The listing builds one solid part. Answer for the finished solid, in the listing's coordinates (mm). A direction names the side the tool comes from. Round coordinates to 2 decimals unless told otherwise and drop trailing zeros. Write each loop counter-clockwise with the first axis right and the second up, starting at its lowest first coordinate (ties: lowest second). Pieces come first, ordered by that corner, then holes. Notation, with made-up numbers: M -11.75,-35 L 46.25,-35 A15 ccw 46.25,-16 Z; hole C 50.5,30 d7. An arc over 180 degrees is marked long. Put each result on its own line as item: value. Start each with the question number.
```python
from build123d import *

# Parameters (mm, degrees)
EXTRUDE1_DEPTH     = 17.78
SKETCH3_R          = 15.08125
SKETCH3_R_2        = 3.4925
SKETCH3_R_3        = 1.5875
CUT_EXTRUDE1_DEPTH = 17.78
CUT_EXTRUDE2_DEPTH = 5.08
SKETCH5_W          = 14.2875
SKETCH5_H          = 404.0251
CUT_EXTRUDE3_DEPTH = 11.43
CUT_EXTRUDE4_DEPTH = 396.08125


with BuildPart() as part:
    # Sketch2 → Extrude1 (new body)
    with BuildSketch(Plane.XY):
        Polygon((11695.641666666, -6048.53375), (11699.451666666, -6052.34375), (12250.631666666, -6052.34375), (12254.441666666, -6048.53375), (12254.441666666, -5656.2625), (11695.641666666, -5656.2625), align=None)
    extrude(amount=-EXTRUDE1_DEPTH)

    # Sketch3 → Cut-Extrude1 (cut)
    with BuildSketch(Plane.XY):
        with Locations((12197.291666666, -5761.0375)):
            Circle(SKETCH3_R)
        with Locations((12138.554166666, -5833.26875)):
            Circle(SKETCH3_R_2)
        with Locations((12196.974166666, -5865.01875)):
            Circle(SKETCH3_R_3)
        with Locations((12196.974166666, -5922.16875)):
            Circle(SKETCH3_R_3)
        with Locations((12196.974166666, -5979.31875)):
            Circle(SKETCH3_R_3)
        with Locations((12140.141666666, -6037.10375)):
            Circle(SKETCH3_R_3)
        with Locations((11975.041666666, -6037.10375)):
            Circle(SKETCH3_R_3)
        with Locations((11809.941666666, -6037.10375)):
            Circle(SKETCH3_R_3)
        with Locations((11753.109166666, -5979.31875)):
            Circle(SKETCH3_R_3)
        with Locations((11753.109166666, -5922.16875)):
            Circle(SKETCH3_R_3)
        with Locations((11753.109166666, -5865.01875)):
            Circle(SKETCH3_R_3)
        with Locations((11811.529166666, -5833.26875)):
            Circle(SKETCH3_R_2)
        with Locations((11975.041666666, -5973.7625)):
            Circle(SKETCH3_R_2)
        with Locations((11975.041666666, -5692.775)):
            Circle(SKETCH3_R_2)
        with BuildLine():
            Line((11841.691666666, -5702.2873), (12108.391666666, -5702.2873))
            ThreePointArc((12108.391666666, -5702.2873), (12122.993563119, -5708.335603547), (12129.041866666, -5722.9375))
            Line((12129.041866666, -5722.9375), (12129.041866666, -5943.6))
            ThreePointArc((12129.041866666, -5943.6), (12122.993563119, -5958.201896453), (12108.391666666, -5964.2502))
            Line((12108.391666666, -5964.2502), (11841.691666666, -5964.2502))
            ThreePointArc((11841.691666666, -5964.2502), (11827.089770213, -5958.201896453), (11821.041466666, -5943.6))
            Line((11821.041466666, -5943.6), (11821.041466666, -5722.9375))
            ThreePointArc((11821.041466666, -5722.9375), (11827.089770213, -5708.335603547), (11841.691666666, -5702.2873))
        make_face()
        with BuildLine():
            Line((11734.654409808, -5693.754968556), (11739.23011943, -5693.754968556))
            ThreePointArc((11739.23011943, -5693.754968556), (11748.029166666, -5687.976468556), (11756.828213901, -5693.754968556))
            Line((11756.828213901, -5693.754968556), (11761.386355753, -5693.754968556))
            ThreePointArc((11761.386355753, -5693.754968556), (11767.531113043, -5692.357368906), (11771.079666666, -5697.564968556))
            ThreePointArc((11771.079666666, -5697.564968556), (11767.531113043, -5702.772568206), (11761.386355753, -5701.374968556))
            Line((11761.386355753, -5701.374968556), (11756.828213901, -5701.374968556))
            ThreePointArc((11756.828213901, -5701.374968556), (11754.760305425, -5704.393665595), (11751.712166666, -5706.417925308))
            Line((11751.712166666, -5706.417925308), (11751.712166666, -5721.30243896))
            ThreePointArc((11751.712166666, -5721.30243896), (11748.029166666, -5731.092968556), (11744.346166666, -5721.30243896))
            Line((11744.346166666, -5721.30243896), (11744.346166666, -5706.417925308))
            ThreePointArc((11744.346166666, -5706.417925308), (11741.298027907, -5704.393665595), (11739.23011943, -5701.374968556))
            Line((11739.23011943, -5701.374968556), (11734.654409809, -5701.374968556))
            ThreePointArc((11734.654409809, -5701.374968556), (11724.978666666, -5697.564968556), (11734.654409808, -5693.754968556))
        make_face()
    extrude(amount=-CUT_EXTRUDE1_DEPTH, mode=Mode.SUBTRACT)

    # Sketch4 → Cut-Extrude2 (cut)
    with BuildSketch(Plane.XY):
        Polygon((11975.041666666, -6028.21375), (11695.641666666, -6028.21375), (11695.641666666, -6045.99375), (12254.441666666, -6045.99375), (12254.441666666, -6028.21375), align=None)
    extrude(amount=-CUT_EXTRUDE2_DEPTH, mode=Mode.SUBTRACT)

    # Sketch5 → Cut-Extrude3 (cut)
    with BuildSketch(Plane.XY):
        with Locations((11694.847916666, -5853.51255)):
            Rectangle(SKETCH5_W, SKETCH5_H)
        with Locations((12255.235416666, -5853.51255)):
            Rectangle(SKETCH5_W, SKETCH5_H)
    extrude(amount=-CUT_EXTRUDE3_DEPTH, mode=Mode.SUBTRACT)

    # Sketch7 → Cut-Extrude4 (cut)
    with BuildSketch(Plane.XZ.offset(6052.34375)):
        Polygon((12254.441666666, -17.78), (12254.441666666, -11.43), (12248.091666666, -11.43), align=None)
        Polygon((11695.641666666, -17.78), (11695.641666666, -11.43), (11701.991666666, -11.43), align=None)
    extrude(amount=-CUT_EXTRUDE4_DEPTH, mode=Mode.SUBTRACT)


solid = part.part
```
Item 1: Which of the six approach directions +Z, -Z, +X, -X, +Y, -Y give full straight-line access (tool end or side, diameter ignored) to faces 1 (the cylindrical face through (11747.873, -5687.978, -8.766)), 2 (the flat face through (11971, -6005, 0)), 3 (the flat face through (12248.092, -5857, -6))?
Item 2: Flat-ended cylindrical pins translate along their axes: pin 1 (5 mm diameter, centred on x = 11975.04, y = -6037.1, fed in from +Z); pin 2 (14.5 mm diameter, centred on x = 11748.03, y = -5725.5, fed in from +Z); pin 3 (1 mm diameter, centred on y = -5909, z = -15.5, fed in from -X); pin 4 (5.5 mm diameter, centred on y = -5822.5, z = -5, fed in from -X). Find the tip coordinate at first contact, or state that the pin passes through.
Item 3: Section B-B (y = -5794) is taken. Give the vertices of the cut face in (x, z).
Item 4: Consider line 1 along Y through (x, z) = (12037, -2.5); line 2 along Y through (x, z) = (11730, -12); line 3 along X through (y, z) = (-5902.5, -6.25). Determine where each line is inside the solid, lowest interval first. Write a range as [from, to].
Item 5: Section A-A (x = 11936) is taken. Give the vertices of the cut face in (y, z), and give its area (3 significant figures).
Item 6: Determine the mould class of faces 4 (the flat face through (11701.992, -5857, -6)), 5 (the flat face through (11971, -5984, -17.78)), 6 (the cylindrical face through (11724.98, -5697.75, -8.77)) for opening direction X: released by +X, released by -X, zero draft, split by the parting line, or undercut.
Item 7: Section D-D (y = -5951) is taken. Give the vertices of the cut face in (x, z), and give its area (3 significant figures).
Item 8: Section C-C (y = -6001) is taken. Give the vertices of the cut face in (x, z).
Output values:
1. face 1: +Z, -Z
1. face 2: +Z, +X, -X, +Y, -Y
1. face 3: +Z, +X, +Y, -Y
2. pin 1: stops at z = -5.08
2. pin 2: stops at z = 0
2. pin 3: stops at x = 11697.42
2. pin 4: stops at x = 11701.99
3. outline: M 11695.64,-17.78 L 11821.04,-17.78 L 11821.04,0 L 11701.99,0 L 11701.99,-11.43 Z; M 12129.04,-17.78 L 12254.44,-17.78 L 12248.09,-11.43 L 12248.09,0 L 12129.04,0 Z
4. line 1: y = [-6052.34, -6045.99], [-6028.21, -5964.25], [-5702.29, -5656.26]
4. line 2: y = [-6052.34, -5703.12], [-5692.01, -5656.26]
4. line 3: x = [11701.99, 11821.04], [12129.04, 12248.09]
5. outline: M -6052.34,-17.78 L -5964.25,-17.78 L -5964.25,0 L -6028.21,0 L -6028.21,-5.08 L -6045.99,-5.08 L -6045.99,0 L -6052.34,0 Z; M -5702.29,-17.78 L -5656.26,-17.78 L -5656.26,0 L -5702.29,0 Z
5. area: 2,290 mm^2
6. face 4: released by -X
6. face 5: zero draft
6. face 6: undercut
7. outline: M 11695.64,-17.78 L 11822.41,-17.78 L 11822.41,0 L 11701.99,0 L 11701.99,-11.43 Z; M 12127.67,-17.78 L 12254.44,-17.78 L 12248.09,-11.43 L 12248.09,0 L 12127.67,0 Z
7. area: 4,320 mm^2
8. outline: M 11695.64,-17.78 L 12254.44,-17.78 L 12248.09,-11.43 L 12248.09,0 L 11701.99,0 L 11701.99,-11.43 Z
